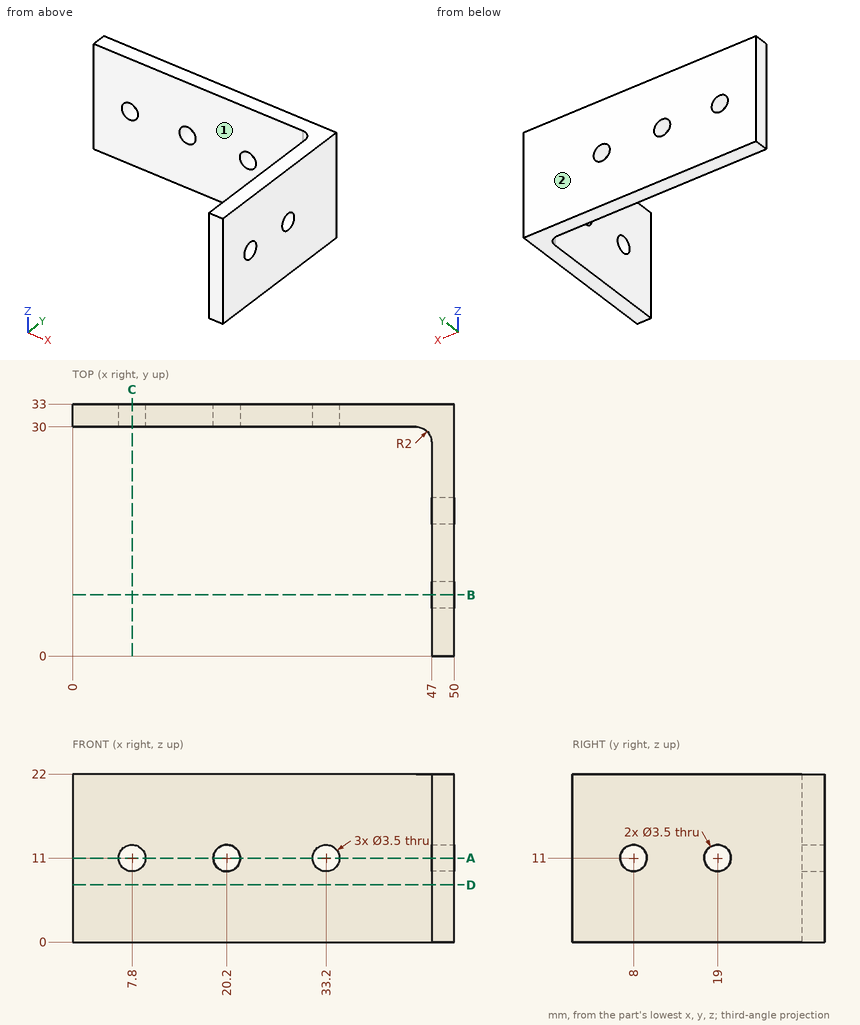
Here's the drawing with two shaded views (mm, measured from the low corner). I have some questions. A direction names the side the tool comes from. Coordinates: 2 decimals unless noted, no trailing zeros. Loops run counter-clockwise (first coordinate to the right, second up) from the corner with the lowest first, then second, coordinate; pieces in that order, holes last.
Item 1: Which directions (+Z, -Z, +X, -X, +Y, -Y) give clear straight access to the entire face, cutting with the end or side of a thin tool? Please do the marked faces 1 and 2.
Answers below:
face 1: +Z, -Z, -X, -Y
face 2: +Z, -Z, +X, -X, +Y
Item 2: Suppose I cut it at B-B (y = 8). Please give me the cut outline in (x, z).
Answers below:
outline: (47, 0) - (50, 0) - (50, 9.25) - (47, 9.25) - close; (47, 12.75) - (50, 12.75) - (50, 22) - (47, 22) - close
Item 3: Please list where these lines run through material, in increasing order: L1, parallel to Y at x = 48.95, z = 11; L2, parallel to X at y = 31.2, z = 11; L3, parallel to Z at x = 49.3, y = 8.
Answers below:
L1: y = 0 to 6.25, 9.75 to 17.25, 20.75 to 33
L2: x = 0 to 6.05, 9.55 to 18.45, 21.95 to 31.45, 34.95 to 50
L3: z = 0 to 9.25, 12.75 to 22
Item 4: I'm going to push flat-ended pins straight in: pin 1 (4 mm diameter, centred on x = 15.5, z = 17.5, fed in from -Y); pin 2 (6 mm diameter, centred on y = 17.5, z = 12.5, fed in from -X); pin 3 (4 mm diameter, centred on x = 20.2, z = 11, fed in from +Y). Where does each tip first touch, or does it pass through?
Answers below:
pin 1: stops at y = 30
pin 2: stops at x = 47
pin 3: stops at y = 33
Item 5: Suppose I cut it at A-A (z = 11). Please give me the cut outline in (x, y).
Answers below:
outline: (0, 30) - (6.05, 30) - (6.05, 33) - (0, 33) - close; (9.55, 30) - (18.45, 30) - (18.45, 33) - (9.55, 33) - close; (21.95, 30) - (31.45, 30) - (31.45, 33) - (21.95, 33) - close; (34.95, 30) - (45, 30) arc R2 cw to (47, 28) - (47, 20.75) - (50, 20.75) - (50, 33) - (34.95, 33) - close; (47, 0) - (50, 0) - (50, 6.25) - (47, 6.25) - close; (47, 9.75) - (50, 9.75) - (50, 17.25) - (47, 17.25) - close
Item 6: Suppose I cut it at C-C (x = 7.8). Please give me the cut outline in (y, z).
Answers below:
outline: (30, 0) - (33, 0) - (33, 9.25) - (30, 9.25) - close; (30, 12.75) - (33, 12.75) - (33, 22) - (30, 22) - close
Item 7: Suppose I cut it at D-D (z = 7.5). Please give me the cut outline in (x, y).
Answers below:
outline: (0, 30) - (45, 30) arc R2 cw to (47, 28) - (47, 0) - (50, 0) - (50, 33) - (0, 33) - close
